Source: CAD feature listing. Evaluate the final solid. Frame: model axes, mm. A direction names the side the tool comes from. Give positions to 0.01 mm unless a question says otherwise; leave off trailing zeros. Order: outer loops, then holes, each group sorted by start corner. A loop starts at its lowest first (then second) coordinate and runs counter-clockwise, first axis right, second up. Notation, with made-up numbers: (13.5, 4) -> (56.5, 4) arc R26 cw to (56.5, 27) -> close; hole circle Ø9 at (-11, 41). An arc over 180 degrees is marked (long way). Answer in a Markdown table with one row per item.
```python
from build123d import *

# Parameters (mm, degrees)
F0_W     = 52.350345999
F0_H     = 45.2565550804
F1_DEPTH = 55
F2_R     = 5
F3_R     = 10.5851243618
F4_DEPTH = 100


with BuildPart() as f1:
    # F0 (on Front) → F1 (new body, symmetric)
    with BuildSketch(Plane.XZ):
        with Locations((26.1751729995, 22.6282775402)):
            Rectangle(F0_W, F0_H)
    extrude(amount=F1_DEPTH, both=True)

    # F2
    f2_edges = [f1.edges().sort_by_distance(p)[0] for p in [
        (52.350346, -55, 22.628278),
        (0, -55, 22.628278),
        (0, 55, 22.628278),
    ]]
    fillet(f2_edges, radius=F2_R)

    # F3 (on face) → F4 (join)
    with BuildSketch(Plane(origin=(0, 0, 0), x_dir=(1, 0, 0), z_dir=(0, 0, -1))):
        with Locations((15.048192814, 17.3339936882)):
            Circle(F3_R)
    extrude(amount=F4_DEPTH)


solid = f1.part
```
(1) Section query C-C (z = -37). Return the cut outline in (x, y).
A:
| item | result |
|---|---|
| outline | circle Ø21.17 at (15.05, -17.33) |
(2) First-contact query: pin 1 Ø2 at (x, z) = (17.5, -23) entering from +Y; pin 2 Ø1.5 at (x, y) = (26, 39) entering from -Z. Flat tips, straight axial feed; report the tip coordinate or a pass-through.
A:
| item | result |
|---|---|
| pin 1 | stops at y = -6.85 |
| pin 2 | stops at z = 0 |
(3) Ray query, probe 1 along Z at (x, y) = (29.5, 23); probe 2 along X at (y, z) = (-27, -55.5); probe 3 along X at (y, z) = (-24, -82.5). Return the intervals inside material, ascending.
A:
| item | result |
|---|---|
| probe 1 | z = 0 to 45.26 |
| probe 2 | x = 10.73 to 19.36 |
| probe 3 | x = 6.83 to 23.27 |
(4) Section query D-D (y = 28). Return the cut outline in (x, z), plus the area to 3 significant figures.
A:
| item | result |
|---|---|
| outline | (0, 0) -> (52.35, 0) -> (52.35, 45.26) -> (0, 45.26) -> close |
| area | 2,370 mm^2 |
(5) Section query A-A (y = -25.5). Return the cut outline in (x, z).
A:
| item | result |
|---|---|
| outline | (0, 0) -> (8.31, 0) -> (8.31, -100) -> (21.78, -100) -> (21.78, 0) -> (52.35, 0) -> (52.35, 45.26) -> (0, 45.26) -> close |
(6) Access query for faces 1 (the cylindrical face through (13.67, -27.83, -49.3)), 2 (the flat face through (28, 55, 23)). Directions: +Z, -Z, +X, -X, +Y, -Y. A direction counts if a zero-diameter tool reaches every point of the face in a straight line with its end or side. Return the directions, or none.
A:
| item | result |
|---|---|
| face 1 | -Z |
| face 2 | +Z, -Z, +X, -X, +Y |
(7) Section query B-B (x = 40.5). Return the cut outline in (y, z), plus the area to 3 significant figures.
A:
| item | result |
|---|---|
| outline | (-55, 0) -> (55, 0) -> (55, 45.26) -> (-55, 45.26) -> close |
| area | 4,980 mm^2 |
